Could you check a few things on this model? Use its own coordinates, in mm. Coordinates: 2 decimals unless noted, no trailing zeros. Loops run counter-clockwise (first coordinate to the right, second up) from the corner with the lowest first, then second, coordinate; pieces in that order, holes last. Notation, with made-up numbers: M -25.75,73 L 15.25,73 A6 ccw 15.25,84 Z; hole C 89.5,35 d2. An arc over 180 degrees is marked long. Return JSON: item names as keys, results as strings. Group by question number.
from build123d import *

# Parameters (mm, degrees)
SKETCH1_W           = 130
SKETCH1_H           = 156
SKETCH1_R           = 3
BOSS_EXTRUDE1_DEPTH = 10
SKETCH2_R           = 2.5
CUT_EXTRUDE1_DEPTH  = 10
SKETCH3_W           = 130
SKETCH3_H           = 10
BOSS_EXTRUDE2_DEPTH = 10
SKETCH4_W           = 130
SKETCH4_H           = 10
CUT_EXTRUDE2_DEPTH  = 10
SKETCH5_W           = 130
SKETCH5_H           = 10
BOSS_EXTRUDE3_DEPTH = 10
SKETCH6_W           = 130
SKETCH6_H           = 10
BOSS_EXTRUDE4_DEPTH = 8.98


with BuildPart() as part:
    # Sketch1 → Boss-Extrude1 (new body)
    with BuildSketch(Plane(origin=(0, 0, 0), x_dir=(1, 0, 0), z_dir=(0, 1, 0))):
        with Locations((65, -43.506875339)):
            Rectangle(SKETCH1_W, SKETCH1_H)
        with Locations(Location((5, 27.493124661, 0), (0, 0, 270))):
            Circle(SKETCH1_R, mode=Mode.SUBTRACT)
        with Locations(Location((45, 27.493124661, 0), (0, 0, 270))):
            Circle(SKETCH1_R, mode=Mode.SUBTRACT)
        with Locations(Location((45, -12.506875339, 0), (0, 0, 270))):
            Circle(SKETCH1_R, mode=Mode.SUBTRACT)
        with Locations(Location((5, -12.506875339, 0), (0, 0, 270))):
            Circle(SKETCH1_R, mode=Mode.SUBTRACT)
        with Locations(Location((85, 27.493124661, 0), (0, 0, 270))):
            Circle(SKETCH1_R, mode=Mode.SUBTRACT)
        with Locations(Location((125, 27.493124661, 0), (0, 0, 270))):
            Circle(SKETCH1_R, mode=Mode.SUBTRACT)
        with Locations(Location((85, -12.506875339, 0), (0, 0, 270))):
            Circle(SKETCH1_R, mode=Mode.SUBTRACT)
        with Locations(Location((125, -12.506875339, 0), (0, 0, 270))):
            Circle(SKETCH1_R, mode=Mode.SUBTRACT)
        with Locations(Location((85, -74.506875339, 0), (0, 0, 270))):
            Circle(SKETCH1_R, mode=Mode.SUBTRACT)
        with Locations(Location((125, -74.506875339, 0), (0, 0, 270))):
            Circle(SKETCH1_R, mode=Mode.SUBTRACT)
        with Locations(Location((125, -114.506875339, 0), (0, 0, 270))):
            Circle(SKETCH1_R, mode=Mode.SUBTRACT)
        with Locations(Location((85, -114.506875339, 0), (0, 0, 270))):
            Circle(SKETCH1_R, mode=Mode.SUBTRACT)
        with Locations(Location((5, -74.506875339, 0), (0, 0, 270))):
            Circle(SKETCH1_R, mode=Mode.SUBTRACT)
        with Locations(Location((45, -74.506875339, 0), (0, 0, 270))):
            Circle(SKETCH1_R, mode=Mode.SUBTRACT)
        with Locations(Location((5, -114.506875339, 0), (0, 0, 270))):
            Circle(SKETCH1_R, mode=Mode.SUBTRACT)
        with Locations(Location((45, -114.506875339, 0), (0, 0, 270))):
            Circle(SKETCH1_R, mode=Mode.SUBTRACT)
    extrude(amount=BOSS_EXTRUDE1_DEPTH)

    # Sketch2 → Cut-Extrude1 (cut)
    with BuildSketch(Plane(origin=(0, 10, 0), x_dir=(1, 0, 0), z_dir=(0, 1, 0))):
        with Locations(Location((98, -31.506875339, 0), (0, 0, 270))):
            Circle(SKETCH2_R)
        with Locations(Location((98, -55.506875339, 0), (0, 0, 270))):
            Circle(SKETCH2_R)
        with Locations(Location((122, -55.506875339, 0), (0, 0, 270))):
            Circle(SKETCH2_R)
        with Locations(Location((122, -31.506875339, 0), (0, 0, 270))):
            Circle(SKETCH2_R)
    extrude(amount=-CUT_EXTRUDE1_DEPTH, mode=Mode.SUBTRACT)

    # Sketch3 → Boss-Extrude2 (add)
    with BuildSketch(Plane(origin=(0, 0, -34.493124661), x_dir=(-1, 0, 0), z_dir=(0, 0, -1))):
        with Locations((-65, 5)):
            Rectangle(SKETCH3_W, SKETCH3_H)
    extrude(amount=BOSS_EXTRUDE2_DEPTH)

    # Sketch4 → Cut-Extrude2 (cut)
    with BuildSketch(Plane(origin=(0, 0, -44.493124661), x_dir=(-1, 0, 0), z_dir=(0, 0, -1))):
        with Locations((-65, 5)):
            Rectangle(SKETCH4_W, SKETCH4_H)
    extrude(amount=-CUT_EXTRUDE2_DEPTH, mode=Mode.SUBTRACT)

    # Sketch5 → Boss-Extrude3 (add)
    with BuildSketch(Plane.XY.offset(121.506875339)):
        with Locations((65, 5)):
            Rectangle(SKETCH5_W, SKETCH5_H)
    extrude(amount=BOSS_EXTRUDE3_DEPTH)

    # Sketch6 → Boss-Extrude4 (add)
    with BuildSketch(Plane(origin=(0, 0, -34.493124661), x_dir=(-1, 0, 0), z_dir=(0, 0, -1))):
        with Locations((-65, 5)):
            Rectangle(SKETCH6_W, SKETCH6_H)
    extrude(amount=BOSS_EXTRUDE4_DEPTH)


solid = part.part
(1) Imagine slicing it at B-B, the plane x = 85. Write out the boundary of the cut face in (y, z).
(2) Will this pin go through, and if not, where does the flat tip stop? P1, Ø8, axis at x = 125, z = 114.51, coming from the +Y side.
(3) We'd pull the mould along X, two halves only. Please class faces 1 (the face through (0, 5, 45)), 2 (the face through (66, 5, -43.473)), 3 (the face through (124.48, 5.07, 55.18)): +X half, -X half, draft (parallel to the pull), parting line (faces both ways), or undercut.
(4) If I drill on L1, parallel to X at y = 8.25, z = 12; L2, parallel to Z at x = 99, y = 4.75; L3, parallel to Z at x = 47.5, y = 7, over which ranges is the centre line in solid material (lowest first)? Write a range as [from, to].
(5) Imagine slicing it at C-C, the plane y = 3.75. Count the separate pieces of the cut face and the enclosed holes in it, then the cut area to 3 significant figures.
(6) Imagine slicing it at A-A, the plane x = 98. Write out the boundary of the cut face in (y, z), then the cut area to 3 significant figures.
Checks:
{
 "1": {"outline": "M 0,-43.47 L 10,-43.47 L 10,-30.49 L 0,-30.49 Z; M 0,-24.49 L 10,-24.49 L 10,9.51 L 0,9.51 Z; M 0,15.51 L 10,15.51 L 10,71.51 L 0,71.51 Z; M 0,77.51 L 10,77.51 L 10,111.51 L 0,111.51 Z; M 0,117.51 L 10,117.51 L 10,131.51 L 0,131.51 Z"},
 "2": {"P1": "y = 10"},
 "3": {"face 1": "-X half", "face 2": "draft", "face 3": "undercut"},
 "4": {"L1": "[0, 2.04], [7.96, 42.04], [47.96, 82.04], [87.96, 122.04], [127.96, 130]", "L2": "[-43.47, 29.22], [33.8, 53.22], [57.8, 131.51]", "L3": "[-43.47, -29.15], [-25.83, 10.85], [14.17, 72.85], [76.17, 112.85], [116.17, 131.51]"},
 "5": {"separate pieces": "1", "enclosed holes": "20", "area": "22,200 mm²"},
 "6": {"outline": "M 0,-43.47 L 10,-43.47 L 10,29.01 L 0,29.01 Z; M 0,34.01 L 10,34.01 L 10,53.01 L 0,53.01 Z; M 0,58.01 L 10,58.01 L 10,131.51 L 0,131.51 Z", "area": "1,650 mm²"}
}
